from build123d import *

# Parameters (mm, degrees)
SKETCH_1_R      = 20
EXTRUDE_1_DEPTH = 170
SKETCH_2_W      = 40
SKETCH_2_H      = 40
EXTRUDE_2_DEPTH = 50
SKETCH_3_W      = 100
SKETCH_3_H      = 30
EXTRUDE_3_DEPTH = 40
SKETCH_4_W      = 100
SKETCH_4_H      = 30
EXTRUDE_4_DEPTH = 40
FILLET_1_R      = 10
EXTRUDE_6_DEPTH = 20
EXTRUDE_7_DEPTH = 20
SKETCH_10_R     = 10
EXTRUDE_8_DEPTH = 20


with BuildPart() as part:
    # 스케치1 → 보스-돌출1 (new body)
    with BuildSketch(Plane.XY):
        Circle(SKETCH_1_R)
    extrude(amount=EXTRUDE_1_DEPTH)

    # 스케치2 → 보스-돌출2 (add)
    with BuildSketch(Plane(origin=(0, 0, 0), x_dir=(0, 0, -1), z_dir=(1, 0, 0))):
        with Locations((-20, 0)):
            Rectangle(SKETCH_2_W, SKETCH_2_H)
        with Locations((-105, 0)):
            Rectangle(SKETCH_2_W, SKETCH_2_H)
    extrude(amount=EXTRUDE_2_DEPTH)

    # 스케치3 → 보스-돌출3 (add)
    with BuildSketch(Plane(origin=(0, 0, 0), x_dir=(-1, 0, 0), z_dir=(0, 0, -1))):
        with Locations((-100, -31)):
            Rectangle(SKETCH_3_W, SKETCH_3_H)
        with Locations((-100, 31)):
            Rectangle(SKETCH_3_W, SKETCH_3_H)
    extrude(amount=-EXTRUDE_3_DEPTH)

    # 스케치4 → 보스-돌출4 (add)
    with BuildSketch(Plane(origin=(0, 0, 85), x_dir=(-1, 0, 0), z_dir=(0, 0, -1))):
        with Locations((-100, -31)):
            Rectangle(SKETCH_4_W, SKETCH_4_H)
        with Locations((-100, 31)):
            Rectangle(SKETCH_4_W, SKETCH_4_H)
    extrude(amount=-EXTRUDE_4_DEPTH)

    # 필렛1
    fillet_1_edges = [part.edges().sort_by_distance(p)[0] for p in [
        (50, -20, 20),
        (50, 20, 105),
        (50, -20, 105),
        (50, -16, 20),
        (50, 16, 20),
        (50, -16, 105),
        (50, 16, 105),
        (50, 20, 20),
    ]]
    fillet(fillet_1_edges, radius=FILLET_1_R)

    # 스케치11 → 보스-돌출6 (add, symmetric)
    with BuildSketch(Plane.XY.offset(20)):
        Polygon((20, 20), (50, 38), (50, 46), (6.666666667, 20), align=None)
        Polygon((20, -20), (50, -38), (50, -46), (6.666666667, -20), align=None)
    extrude(amount=EXTRUDE_6_DEPTH, both=True)

    # 스케치13 → 보스-돌출7 (add, symmetric)
    with BuildSketch(Plane.XY.offset(105)):
        Polygon((20, 20), (50, 38), (50, 46), (6.666666667, 20), align=None)
        Polygon((20, -20), (6.666666667, -20), (50, -46), (50, -38), align=None)
    extrude(amount=EXTRUDE_7_DEPTH, both=True)

    # 스케치10 → 보스-돌출8 (add)
    with BuildSketch(Plane.XY.offset(170)):
        Circle(SKETCH_10_R)
    extrude(amount=EXTRUDE_8_DEPTH)


solid = part.part
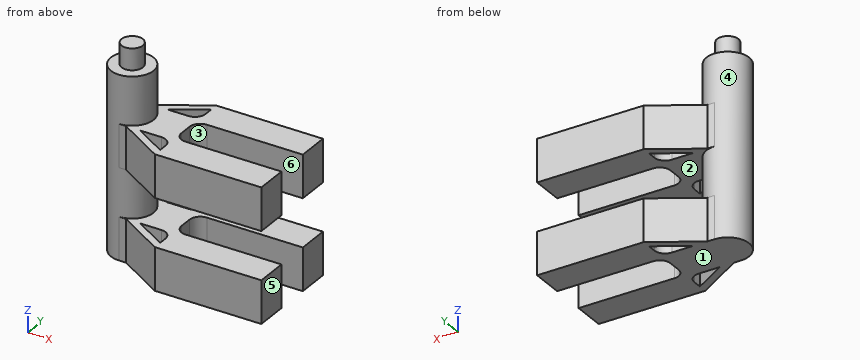
The listing builds one solid part. Answer for the finished solid, in the listing's coordinates (mm). Face numbers are marked on the shaded views. A direction names the side the tool comes from. Round coordinates to 2 decimals unless told otherwise and drop trailing zeros. Write each loop counter-clockwise with the first axis right and the second up, starting at its lowest first coordinate (ties: lowest second). Pieces come first, ordered by that corner, then holes. Notation, with made-up numbers: M 61.25,59.25 L 87.25,59.25 A25 ccw 87.25,89.25 Z; hole C -27.5,52 d3. An arc over 180 degrees is marked long. Write each question's results on one line, items separated by ' | '. Start each with the question number.
Item 1: Straight lines are drawn through the part: L1, parallel to Y at x = 81, z = 13; L2, parallel to Z at x = 103, y = -30.5; L3, parallel to Z at x = -5.5, y = -12.5. For each, find the intervals that lie inside material, in ascending order. Write a range as [from, to].
Item 2: A cutting plane is placed at A-A on z = 25. Write down the section's boundary in (x, y).
Item 3: For the marked faces 4, 5 and 6, determine the directions among +Z, -Z, +X, -X, +Y, -Y from which every point of the face is accessible in a straight line to the end or side of a thin tool.
Item 4: For a pull along Z with two mould halves and no side action, classify the marked faces 1, 2 and 3 as pulls with the +Z half, pulls with the -Z half, needs draft (parallel to the pull), parting line crosses it, or undercut.
Item 5: Flat-ended cylindrical pins translate along their axes: pin 1 Ø6.5 at (y, z) = (-35, 106.5) entering from -X; pin 2 Ø16 at (x, z) = (29, 96.5) entering from +Y; pin 3 Ø2 at (x, z) = (4.5, 30) entering from +Y. Find the tip coordinate at first contact, or state that the pin passes through.
Item 6: A cutting plane is placed at B-B on y = 0. Write down the section's boundary in (x, z), and give its area (3 significant figures).
Item 7: A cutting plane is placed at C-C on y = -33. Write down the section's boundary in (x, z).
Item 8: A cutting plane is placed at D-D on x = 13.5. Write down the section's boundary in (y, z).
Check sheet entries:
1) L1: [-46, -16], [16, 46] | L2: [0, 40], [85, 125] | L3: [0, 170]
2) outline: M 0,-20 L 6.67,-20 L 50,-46 L 150,-46 L 150,-16 L 60,-16 A10 cw 50,-6 L 50,6 A10 cw 60,16 L 150,16 L 150,46 L 50,46 L 6.67,20 L 0,20 A20 ccw Z; hole M 20,-20 L 50,-38 L 50,-30 A10 ccw 40,-20 Z; hole M 20,20 L 40,20 A10 ccw 50,30 L 50,38 Z
3) face 4: none | face 5: +Z, -Z, +X, +Y, -Y | face 6: +Z, -Z, +X
4) face 1: pulls with the -Z half | face 2: undercut | face 3: needs draft
5) pin 1: x = 26.25 | pin 2: y = 38.2 | pin 3: y = 20
6) outline: M -20,0 L 50,0 L 50,40 L 20,40 L 20,85 L 50,85 L 50,125 L 20,125 L 20,170 L 10,170 L 10,190 L -10,190 L -10,170 L -20,170 Z | area: 9,600 mm²
7) outline: M 28.33,0 L 41.67,0 L 41.67,40 L 28.33,40 Z; M 28.33,85 L 41.67,85 L 41.67,125 L 28.33,125 Z; M 50,0 L 150,0 L 150,40 L 50,40 Z; M 50,85 L 150,85 L 150,125 L 50,125 Z
8) outline: M -24.1,0 L 24.1,0 L 24.1,40 L 14.76,40 L 14.76,85 L 24.1,85 L 24.1,125 L 14.76,125 L 14.76,170 L -14.76,170 L -14.76,125 L -24.1,125 L -24.1,85 L -14.76,85 L -14.76,40 L -24.1,40 Z
